from build123d import *

# Parameters (mm, degrees)
SKETCH1_W                   = 38.1
SKETCH1_H                   = 9.525
BOSS_EXTRUDE1_DEPTH         = 19.05
SKETCH2_W                   = 19.05
SKETCH2_H                   = 6.35
CUT_EXTRUDE1_DEPTH          = 43.8625
F_1_4_0_25_DIAMETER_HOLE2_D = 6.35
CUT_EXTRUDE2_DEPTH          = 31.75


with BuildPart() as part:
    # Sketch1 → Boss-Extrude1 (new, symmetric)
    with BuildSketch(Plane.XY):
        Rectangle(SKETCH1_W, SKETCH1_H)
    extrude(amount=BOSS_EXTRUDE1_DEPTH, both=True)

    # Sketch2 → Cut-Extrude1 (cut, through all)
    with BuildSketch(Plane.XY.offset(19.05)):
        with Locations((9.525, 1.5875)):
            Rectangle(SKETCH2_W, SKETCH2_H)
    extrude(amount=-CUT_EXTRUDE1_DEPTH, mode=Mode.SUBTRACT)

    # 1/4 (0.25) Diameter Hole2 (through all)
    with Locations(Plane(origin=(0, -1.5875, 0), x_dir=(1, 0, 0), z_dir=(0, 1, 0))):
        with Locations((12.7, 12.7), (12.7, -12.7)):
            Hole(F_1_4_0_25_DIAMETER_HOLE2_D / 2)

    # Sketch11 → Cut-Extrude2 (cut)
    with BuildSketch(Plane(origin=(0, 4.7625, 0), x_dir=(1, 0, 0), z_dir=(0, 1, 0))):
        with BuildLine():
            Line((-13.335, -12.7), (-13.335, 12.7))
            ThreePointArc((-13.335, 12.7), (-10.16, 15.875), (-6.985, 12.7))
            Line((-6.985, 12.7), (-6.985, -12.7))
            ThreePointArc((-6.985, -12.7), (-10.16, -15.875), (-13.335, -12.7))
        make_face()
    extrude(amount=-CUT_EXTRUDE2_DEPTH, mode=Mode.SUBTRACT)


solid = part.part
Model file for the job. Use its own axes, mm. A direction names the side the tool comes from. Give positions to 0.01 mm unless a question says otherwise; leave off trailing zeros. Loops run counter-clockwise (first coordinate to the right, second up) from the corner with the lowest first, then second, coordinate; pieces in that order, holes last.
1) Saw through at C-C (y = -1). Write the cut outline in (x, z) (3 decimals), plus the area to 3 significant figures.
2) Saw through at D-D (y = -3.75). Write the cut outline in (x, z) (3 decimals), plus the area to 3 significant figures.
3) Wall check: line 1 (X direction, y = -3, z = 12.7) (3 decimals); line 2 (Z direction, x = 12.7, y = -3) (3 decimals); line 3 (X direction, y = -2, z = -14.5). Give the ranges that are in metal, low to high.
4) Pull direction X, two halves, no side cores. Call faces 1 (the flat face through (-19.05, 0, 0)), 2 (the flat face through (-14, 4.762, 0)), 3 (the cylindrical face through (-10.23, 0.067, -15.874)), 4 (the flat face through (-6.985, 0, 0)): +X half, -X half, draft (parallel to the pull), parting line (faces both ways), or undercut.
5) Tool access for faces 5 (the flat face through (-5, -1, 19.05)), 6 (the flat face through (-13.335, 0, 0)), 7 (the flat face through (9, -1.588, 0)): list every direction of +Z, -Z, +X, -X, +Y, -Y with a clear straight run to the whole face (end or side of a thin tool).
6) Saw through at A-A (x = 12.7). Count the separate pieces of the cut face and the enclosed holes in it, plus the area to 3 significant figures.
7) Flat gauge pins, fed straight in: pin 1 Ø3 at (y, z) = (1.5, -4) entering from +X; pin 2 Ø15 at (x, z) = (10, 4) entering from +Y. Where does each tip first touch, or does it go through?
Answer block:
1. outline: (-19.05, -19.05) - (0, -19.05) - (0, 19.05) - (-19.05, 19.05) - close; hole (-13.335, -12.7) arc R3.175 ccw to (-6.985, -12.7) - (-6.985, 12.7) arc R3.175 ccw to (-13.335, 12.7) - close
1. area: 533 mm2
2. outline: (-19.05, -19.05) - (19.05, -19.05) - (19.05, 19.05) - (-19.05, 19.05) - close; hole (-13.335, -12.7) arc R3.175 ccw to (-6.985, -12.7) - (-6.985, 12.7) arc R3.175 ccw to (-13.335, 12.7) - close; hole circle Ø6.35 at (12.7, -12.7); hole circle Ø6.35 at (12.7, 12.7)
2. area: 1,200 mm2
3. line 1: x = -19.05 to -13.335, -6.985 to 9.525, 15.875 to 19.05
3. line 2: z = -19.05 to -15.875, -9.525 to 9.525, 15.875 to 19.05
3. line 3: x = -19.05 to -12.78, -7.54 to 10.08, 15.32 to 19.05
4. face 1: -X half
4. face 2: draft
4. face 3: undercut
4. face 4: undercut
5. face 5: +Z, +X, -X, +Y, -Y
5. face 6: +Y, -Y
5. face 7: +Z, -Z, +X, +Y
6. separate pieces: 3
6. enclosed holes: 0
6. area: 80.6 mm2
7. pin 1: stops at x = 0
7. pin 2: stops at y = -1.59
